from build123d import *

# Parameters (mm, degrees)
SKETCH_1_R               = 2
EXTRUDE_1_DEPTH          = 10
EXTRUDE_START            = -15
EXTRUDE_2_DEPTH          = 15
EXTRUDE_START_2          = -55
EXTRUDE_3_DEPTH          = 40
CUT_EXTRUDE_1_DEPTH      = 71.775419462
CUT_EXTRUDE_1_DEPTH_BACK = 71.775419462
SKETCH_2_R               = 1.7
SKETCH_2_W               = 6
SKETCH_2_H               = 5.749756634


with BuildPart() as part:
    # 草图1 → 凸台-拉伸1 (new body)
    # profile 1 of 3: a face of its own
    with BuildSketch(Plane.XY):
        with BuildLine():
            Line((3.775539923, 4.499513268), (11.6217341, 13.850243366))
            ThreePointArc((11.6217341, 13.850243366), (12.112655804, 17.579163916), (8.940578549, 19.6))
            Line((8.940578549, 19.6), (-8, 19.6))
            Line((-8, 19.6), (-8, -19.6))
            Line((-8, -19.6), (8.940578549, -19.6))
            ThreePointArc((8.940578549, -19.6), (12.112655804, -17.579163916), (11.6217341, -13.850243366))
            Line((11.6217341, -13.850243366), (3.775539923, -4.499513268))
            ThreePointArc((3.775539923, -4.499513268), (2.137851025, 0), (3.775539923, 4.499513268))
        make_face()
    # profile 2 of 3: a face of its own
    with BuildSketch(Plane.XY):
        with BuildLine():
            Line((-8, -19.6), (-8, 19.6))
            Line((-8, 19.6), (-21.5, 19.6))
            Line((-21.5, 19.6), (-36, 19.6))
            ThreePointArc((-36, 19.6), (-40, 15.6), (-36, 11.6))
            Line((-36, 11.6), (-27.6, 11.6))
            ThreePointArc((-27.6, 11.6), (-16, 0), (-27.6, -11.6))
            Line((-27.6, -11.6), (-36, -11.6))
            ThreePointArc((-36, -11.6), (-40, -15.6), (-36, -19.6))
            Line((-36, -19.6), (-21.5, -19.6))
            Line((-21.5, -19.6), (-8, -19.6))
        make_face()
        with Locations((-36, -15.6)):
            Circle(SKETCH_1_R, mode=Mode.SUBTRACT)
        with Locations((-36, 15.6)):
            Circle(SKETCH_1_R, mode=Mode.SUBTRACT)
    # profile 3 of 3: a face of its own
    with BuildSketch(Plane.XY):
        with BuildLine():
            ThreePointArc((18.601156804, 13.619370123), (15.167616283, 15.432881266), (11.6217341, 13.850243366))
            ThreePointArc((11.6217341, 13.850243366), (12.112655804, 17.579163916), (8.940578549, 19.6))
            Line((8.940578549, 19.6), (20.071646816, 19.6))
            ThreePointArc((20.071646816, 19.6), (28.054072893, 0), (20.071646816, -19.6))
            Line((20.071646816, -19.6), (8.940578549, -19.6))
            ThreePointArc((8.940578549, -19.6), (12.112655804, -17.579163916), (11.6217341, -13.850243366))
            ThreePointArc((11.6217341, -13.850243366), (15.167616283, -15.432881266), (18.601156804, -13.619370123))
            ThreePointArc((18.601156804, -13.619370123), (23.054072893, 0), (18.601156804, 13.619370123))
        make_face()
    extrude(amount=EXTRUDE_1_DEPTH)

    # 草图1<3> → 凸台-拉伸2 (add)
    with BuildSketch(Plane.XY.offset(EXTRUDE_START)):
        with BuildLine():
            Line((3.775539923, 4.499513268), (11.6217341, 13.850243366))
            ThreePointArc((11.6217341, 13.850243366), (12.112655804, 17.579163916), (8.940578549, 19.6))
            Line((8.940578549, 19.6), (-8, 19.6))
            Line((-8, 19.6), (-8, -19.6))
            Line((-8, -19.6), (8.940578549, -19.6))
            ThreePointArc((8.940578549, -19.6), (12.112655804, -17.579163916), (11.6217341, -13.850243366))
            Line((11.6217341, -13.850243366), (3.775539923, -4.499513268))
            ThreePointArc((3.775539923, -4.499513268), (2.137851025, 0), (3.775539923, 4.499513268))
        make_face()
    extrude(amount=EXTRUDE_2_DEPTH)

    # 草图1<4> → 凸台-拉伸3 (add)
    with BuildSketch(Plane.XY.offset(EXTRUDE_START_2)):
        with BuildLine():
            Line((3.775539923, 4.499513268), (11.6217341, 13.850243366))
            ThreePointArc((11.6217341, 13.850243366), (12.112655804, 17.579163916), (8.940578549, 19.6))
            Line((8.940578549, 19.6), (-8, 19.6))
            Line((-8, 19.6), (-8, -19.6))
            Line((-8, -19.6), (8.940578549, -19.6))
            ThreePointArc((8.940578549, -19.6), (12.112655804, -17.579163916), (11.6217341, -13.850243366))
            Line((11.6217341, -13.850243366), (3.775539923, -4.499513268))
            ThreePointArc((3.775539923, -4.499513268), (2.137851025, 0), (3.775539923, 4.499513268))
        make_face()
    extrude(amount=EXTRUDE_3_DEPTH)

    # 草图2 → 切除-拉伸1 (cut, two sides: drawn at the far end of the back side and taken through both)
    with BuildSketch(Plane(origin=(0, 0, 0), x_dir=(0, 0, -1), z_dir=(1, 0, 0)).offset(-CUT_EXTRUDE_1_DEPTH_BACK)):
        with Locations((-5, 0)):
            Circle(SKETCH_2_R)
        with Locations((52, 16.725121683)):
            Rectangle(SKETCH_2_W, SKETCH_2_H)
        with Locations((52, -16.725121683)):
            Rectangle(SKETCH_2_W, SKETCH_2_H)
    extrude(amount=CUT_EXTRUDE_1_DEPTH + CUT_EXTRUDE_1_DEPTH_BACK, mode=Mode.SUBTRACT)


solid = part.part
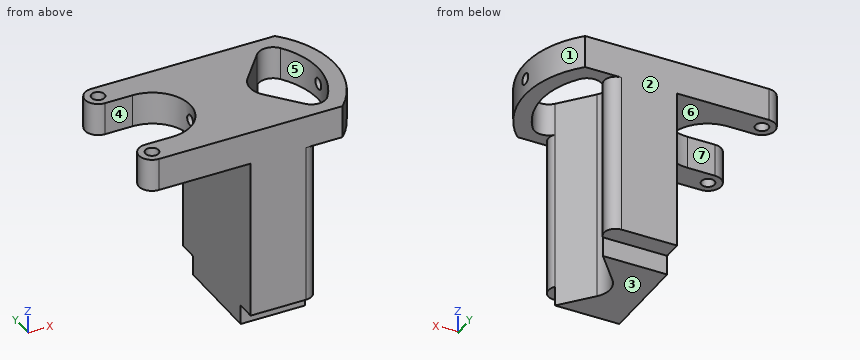
Read the model definition and answer for the solid it produces. Units are mm, in the model's axes. Face numbers are marked on the shaded views. A direction names the side the tool comes from. Coordinates: 2 decimals unless noted, no trailing zeros. Loops run counter-clockwise (first coordinate to the right, second up) from the corner with the lowest first, then second, coordinate; pieces in that order, holes last. Notation, with made-up numbers: (88.25, 60) - (101.25, 60) arc R22 ccw to (101.25, 88) - close; hole circle Ø7 at (61, 71.25). An arc over 180 degrees is marked (long way). Answer in a Markdown table with one row per item.
Q1. For the marked faces 5, 6 and 7, determine the directions among +Z, -Z, +X, -X, +Y, -Y from which every point of the face is accessible in a straight line to the end or side of a thin tool.
Here are the results:
| item | result |
|---|---|
| face 5 | +Z, -Z |
| face 6 | -Z, -X, +Y, -Y |
| face 7 | +Z, -Z, -X |
Q2. Find section C-C on x = 17.5. Write down the section's boundary in (y, z).
Here are the results:
| item | result |
|---|---|
| outline | (-19.6, 0) - (-14.68, 0) - (-14.68, 10) - (-19.6, 10) - close; (14.68, 0) - (19.6, 0) - (19.6, 10) - (14.68, 10) - close |
Q3. Find section A-A on y = 0. Write down the section's boundary in (x, z).
Here are the results:
| item | result |
|---|---|
| outline | (-16, 0) - (-8, 0) - (-8, -55) - (2.14, -55) - (2.14, 3.3) - (-16, 3.3) - close; (-16, 6.7) - (2.14, 6.7) - (2.14, 10) - (-16, 10) - close; (23.05, 0) - (28.05, 0) - (28.05, 3.3) - (23.05, 3.3) - close; (23.05, 6.7) - (28.05, 6.7) - (28.05, 10) - (23.05, 10) - close |
Q4. Given P1, Ø10, axis at y = 8.5, z = -10, coming from the +X side; P2, Ø6.5, axis at x = 5.5, z = -53.5, coming from the -Y side; P3, Ø2, axis at y = 13.5, z = -29.5, coming from the +X side; P4, Ø2.5, axis at x = -36, y = 15.6, coming from the -Z side, each flat-ended and moving along its own axis, determine where each tip first touches the part or whether it passes through.
Here are the results:
| item | result |
|---|---|
| P1 | stops at x = 11.33 |
| P2 | stops at y = -13.85 |
| P3 | stops at x = 12.05 |
| P4 | passes through |
Q5. Straight lines are drawn through the part: line 1 along Y through (x, z) = (-36, 7.5); line 2 along Y through (x, z) = (-5, 5); line 3 along Z through (x, y) = (24.5, 0). For each, find the intervals that lie inside material, in ascending order. Write a range as [from, to].
Here are the results:
| item | result |
|---|---|
| line 1 | y = [-19.6, -17.6], [-13.6, -11.6], [11.6, 13.6], [17.6, 19.6] |
| line 2 | y = [-19.6, -1.7], [1.7, 19.6] |
| line 3 | z = [0, 3.3], [6.7, 10] |
Q6. Find section D-D on z = 5. Write down the section's boundary in (x, y), plus the area to 3 significant figures.
Here are the results:
| item | result |
|---|---|
| outline | (-36, -19.6) - (20.07, -19.6) arc R28.05 ccw to (28, -1.7) - (22.99, -1.7) arc R23.05 cw to (18.6, -13.62) arc R4.44 cw to (11.62, -13.85) - (3.78, -4.5) arc R7 cw to (2.35, -1.7) - (-16.13, -1.7) arc R11.6 cw to (-27.6, -11.6) - (-36, -11.6) arc R4 ccw to start; (-36, 11.6) - (-27.6, 11.6) arc R11.6 cw to (-16.13, 1.7) - (2.35, 1.7) arc R7 cw to (3.78, 4.5) - (11.62, 13.85) arc R4.44 cw to (18.6, 13.62) arc R23.05 cw to (22.99, 1.7) - (28, 1.7) arc R28.05 ccw to (20.07, 19.6) - (-36, 19.6) arc R4 ccw to start; hole circle Ø4 at (-36, -15.6); hole circle Ø4 at (-36, 15.6) |
| area | 1,510 mm^2 |
Q7. The mould has two halves that part along Y. Classify the marked faces 1, 2, 3 and 4: pulls with the +Y half, pulls with the -Y half, needs draft (parallel to the pull), parting line crosses it, or undercut.
Here are the results:
| item | result |
|---|---|
| face 1 | parting line crosses it |
| face 2 | pulls with the +Y half |
| face 3 | needs draft |
| face 4 | undercut |
Q8. Find section B-B on z = -25. Write down the section's boundary in (x, y), plus the area to 3 significant figures.
Here are the results:
| item | result |
|---|---|
| outline | (-8, -19.6) - (8.94, -19.6) arc R3.5 ccw to (11.62, -13.85) - (3.78, -4.5) arc R7 cw to (3.78, 4.5) - (11.62, 13.85) arc R3.5 ccw to (8.94, 19.6) - (-8, 19.6) - close |
| area | 618 mm^2 |
